Here's the drawing with two shaded views (mm, measured from the low corner). I have some questions. Coordinates: 2 decimals unless noted, no trailing zeros. Loops run counter-clockwise (first coordinate to the right, second up) from the corner with the lowest first, then second, coordinate; pieces in that order, holes last. Notation, with made-up numbers: (41, -28) -> (50, -28) arc R22 cw to (50, -17) -> close; hole circle Ø3 at (24, 51.5). An arc over 180 degrees is marked (long way). Answer as a JSON object with one key per item and string values. Group by question number.
Q1. I want a section at A-A on y = 0.5. Write out the boundary of the cut face in (x, z) (3 decimals).
Q2. I need wall thicknesses on line 1 (X direction, y = 2.35, z = 120.5) (3 decimals). Which ranges of the line are inside material? Lowest first, please.
Q3. I want a section at B-B on z = 33. Write out the boundary of the cut face in (x, y) (3 decimals).
Q4. I'm going to push flat-ended pins straight in: pin 1 (1.6 mm diameter, centred on x = 254.5, y = 1, fed in from -Z); pin 2 (1 mm diameter, centred on y = 1.5, z = 14.5, fed in from +X) (3 decimals); pin 3 (1.5 mm diameter, centred on y = 2.5, z = 106, fed in from -X) (3 decimals); pin 4 (4 mm diameter, centred on x = 71.5, z = 43.5, fed in from -Y). Where does each tip first touch, or does it pass through?
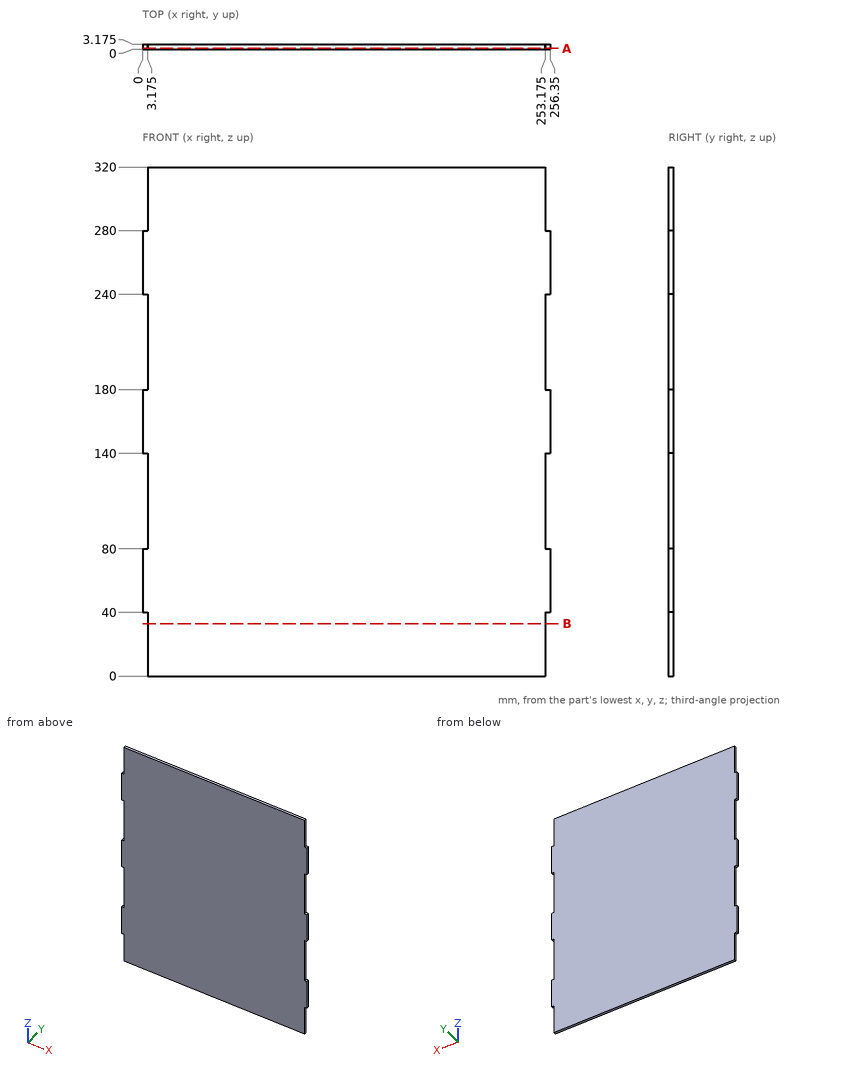
Result set:
{
 "1": {"outline": "(0, 40) -> (3.175, 40) -> (3.175, 0) -> (253.175, 0) -> (253.175, 40) -> (256.35, 40) -> (256.35, 80) -> (253.175, 80) -> (253.175, 140) -> (256.35, 140) -> (256.35, 180) -> (253.175, 180) -> (253.175, 240) -> (256.35, 240) -> (256.35, 280) -> (253.175, 280) -> (253.175, 320) -> (3.175, 320) -> (3.175, 280) -> (0, 280) -> (0, 240) -> (3.175, 240) -> (3.175, 180) -> (0, 180) -> (0, 140) -> (3.175, 140) -> (3.175, 80) -> (0, 80) -> close"},
 "2": {"line 1": "x = 3.175 to 253.175"},
 "3": {"outline": "(3.175, 0) -> (253.175, 0) -> (253.175, 3.175) -> (3.175, 3.175) -> close"},
 "4": {"pin 1": "stops at z = 40", "pin 2": "stops at x = 253.175", "pin 3": "stops at x = 3.175", "pin 4": "stops at y = 0"}
}
